Autodesk Inventor part; units mm, degrees
ref_plane "YZ Plane" through (0, 0, 0) normal (1, 0, 0) x (0, 1, 0)
ref_plane "XZ Plane" through (0, 0, 0) normal (0, 1, 0) x (-1, 0, 0)
ref_plane "XY Plane" through (0, 0, 0) normal (0, 0, 1) x (1, 0, 0)
sketch "Sketch1" plane through (0, 0, 0) normal (1, 0, 0) x (0, 1, 0)
  line L0 (0, 0) -> (50, 0)
  line L1 (50, 0) -> (50, 20)
  line L2 (50, 20) -> (0, 20)
  line L3 (0, 20) -> (0, 0)
  dimension "d0" = 50
  dimension "d1" = 20
extrude "Extrusion1" add sketch "Sketch1" along normal blind 5
sketch "Sketch2" plane through (5, 0, 0) normal (1, 0, 0) x (0, 0, -1)
  line L0 (-20, 50) -> (-20, 0)
  line L1 (-20, 25) -> (0, 25)
  line L2 (0, 0) -> (0, 50)
  line L3 (-20, 20) -> (0, 20)
  line L4 (0, 50) -> (-20, 50) construction
  line L5 (-10, 50) -> (-10, 0) construction
  line L6 (-20, 0) -> (0, 0) construction
  circle A0 centre (-10, 37.5) radius 2.6
  circle A1 centre (-10, 12.5) radius 2.6
  circle A2 centre (-10, 37.5) radius 4.625 construction
  circle A3 centre (-10, 12.5) radius 4.625 construction
  line L7 (-20, 25) -> (-16.5, 25)
  line L8 (-16.5, 25) -> (-16.5, 50)
  line L9 (-16.5, 50) -> (-20, 50)
  line L10 (-20, 50) -> (-20, 25)
  line L11 (0, 25) -> (-3.5, 25)
  line L12 (-3.5, 25) -> (-3.5, 50)
  line L13 (-3.5, 50) -> (0, 50)
  line L14 (0, 50) -> (0, 25)
  line L15 (-20, 20) -> (-16.5, 20)
  line L16 (-16.5, 20) -> (-16.5, 0)
  line L17 (-16.5, 0) -> (-20, 0)
  line L18 (-20, 0) -> (-20, 20)
  line L19 (0, 20) -> (-3.5, 20)
  line L20 (-3.5, 20) -> (-3.5, 0)
  line L21 (-3.5, 0) -> (0, 0)
  line L22 (0, 0) -> (0, 20)
  dimension "d4" = 5
  dimension "d5" = 5.2
  dimension "d6" = 5.2
  dimension "d7" = 12.5
  dimension "d8" = 12.5
  dimension "d9" = 9.25
  dimension "d10" = 9.25
  dimension "d11" = 3.5
  dimension "d12" = 3.5
  dimension "d13" = 3.5
  dimension "d14" = 3.5
extrude "Extrusion2" add sketch "Sketch2" along normal blind 49 contours L9 L8 L1 L0 | L1 L2 L3 L0 | L3 L16 L17 L0 | L12 L13 L2 L1 | L3 L2 L21 L20
chamfer "Chamfer1" distance 25 distance2 27 1 edges at (54, 50, 1.75) measured on face at (54, 23.3333, 18.8333)
chamfer "Chamfer2" distance 25 distance2 27 1 edges at (54, 50, 18.25) measured on face at (54, 23.3333, 18.8333)
chamfer "Chamfer3" distance 20 distance2 27 1 edges at (54, 0, 18.25) measured on face at (54, 15, 18.8333)
chamfer "Chamfer4" distance 20 distance2 27 1 edges at (54, 0, 1.75) measured on face at (54, 15, 1.1667)
sketch "Sketch3" plane through (54, 0, 0) normal (1, 0, 0) x (0, 0, -1)
  line L0 (0, 20) -> (-3.5, 20)
  line L1 (0, 20) -> (0, 25)
  line L2 (-3.5, 25) -> (0, 25)
  line L3 (-3.5, 25) -> (-16.5, 25)
  line L4 (-20, 25) -> (-16.5, 25)
  line L5 (-20, 25) -> (-20, 20)
  line L6 (-16.5, 20) -> (-20, 20)
  line L7 (-16.5, 20) -> (-3.5, 20)
  point P0 (0, 0)
extrude "Extrusion3" add sketch "Sketch3" along normal blind 83
sketch "Sketch4" plane through (5, 25, 16.5) normal (0, 1, 0) x (1, 0, 0)
  line L0 (132, -3.5) -> (132, 16.5)
  line L1 (132, 9) -> (34, 9)
  line L2 (34, 9) -> (34, 4)
  line L3 (34, 4) -> (132, 4)
  line L4 (132, 4) -> (132, 9)
  line L5 (49, 16.5) -> (132, 16.5)
  point P0 (-5, 16.5)
  dimension "d31" = 98
  dimension "d32" = 5
  dimension "d33" = 7.5
extrude "Extrusion4" add sketch "Sketch4" along normal blind 5
sketch "Sketch5" plane through (5, 20, 3.5) normal (0, -1, 0) x (1, 0, 0)
  line L0 (34, 9) -> (34, 4)
  line L1 (132, 9) -> (34, 9)
  line L2 (34, 4) -> (132, 4)
  line L3 (132, 16.5) -> (132, -3.5)
  point P0 (-5, -3.5)
extrude "Extrusion5" add sketch "Sketch5" along normal blind 5
chamfer "Chamfer5" distance 15 distance2 5 1 edges at (137, 30, 10) measured on face at (104.3333, 30, 10.8333)
chamfer "Chamfer6" distance 15 distance2 5 1 edges at (39, 30, 10) measured on face at (94.3333, 30, 10.8333)
chamfer "Chamfer7" distance 15 distance2 5 1 edges at (137, 15, 10) measured on face at (104.3333, 15, 9.1667)
chamfer "Chamfer8" distance 15 distance2 5 1 edges at (39, 15, 10) measured on face at (94.3333, 15, 9.1667)
sketch "Sketch6" plane through (5, 0, 0) normal (1, 0, 0) x (0, 0, -1)
  line L0 (-3.5, 50) -> (-16.5, 50) construction
  line L1 (-10, 50) -> (-10, 0) construction
  line L2 (-20, 0) -> (0, 0) construction
  circle A0 centre (-10, 37.5) radius 2.6
  circle A1 centre (-10, 12.5) radius 2.6
  dimension "d50" = 5.2
  dimension "d51" = 5.2
  dimension "d52" = 12.5
  dimension "d53" = 12.5
extrude "Extrusion6" cut sketch "Sketch6" against normal up to next
sketch "Sketch7" plane through (0, 0, 20) normal (0, 0, 1) x (1, 0, 0)
  line L0 (39, 20) -> (137, 20)
  line L1 (39, 25) -> (137, 25)
  line L2 (137, 20) -> (73, 20)
  line L3 (73, 20) -> (73, 25)
  line L4 (73, 25) -> (137, 25)
  line L5 (137, 25) -> (137, 20)
  point P0 (0, 0)
  point P1 (73, 20)
  dimension "d56" = 64
extrude "Extrusion7" add sketch "Sketch7" along normal blind 20.7
sketch "Sketch8" plane through (5, 25, 16.5) normal (0, 1, 0) x (1, 0, 0)
  line L0 (68, -3.5) -> (68, -24.2)
  line L1 (68, -24.2) -> (132, -24.2)
  line L2 (132, -24.2) -> (132, 3.8)
  line L3 (132, 3.8) -> (68, 3.8)
  line L4 (68, 3.8) -> (68, -24.2)
  line L5 (72, -20.7) -> (128, -20.7) construction
  line L6 (128, -20.7) -> (128, 0.3) construction
  line L7 (128, 0.3) -> (72, 0.3) construction
  line L8 (72, 0.3) -> (72, -20.7) construction
  circle A0 centre (72, -20.7) radius 2.6
  circle A1 centre (72, 0.3) radius 2.6
  circle A2 centre (128, -20.7) radius 2.6
  circle A3 centre (128, 0.3) radius 2.6
  point P0 (-5, 16.5)
  dimension "d59" = 64
  dimension "d60" = 28
  dimension "d61" = 56
  dimension "d62" = 21
  dimension "d63" = 3.5
  dimension "d64" = 4
  dimension "d65" = 5.2
  dimension "d66" = 5.2
  dimension "d67" = 5.2
  dimension "d68" = 5.2
extrude "Extrusion8" cut sketch "Sketch8" against normal up to next contours A0 | A1 | A2 | A3
sketch "Sketch9" plane through (5, 20, 3.5) normal (0, -1, 0) x (1, 0, 0)
  line L0 (68, 37.2) -> (132, 37.2)
  line L1 (117, 9) -> (49, 9)
  line L2 (102.5, 37.2) -> (97.5, 37.2)
  line L3 (97.5, 37.2) -> (97.5, 9)
  line L4 (97.5, 9) -> (102.5, 9)
  line L5 (102.5, 9) -> (102.5, 37.2)
  line L6 (132, 9) -> (132, 37.2)
  point P0 (-5, -3.5)
  point P1 (102.5, 9)
  dimension "d71" = 5
  dimension "d72" = 29.5
extrude "Extrusion9" add sketch "Sketch9" along normal blind 5
chamfer "Chamfer9" distance 15 distance2 5 1 edges at (105, 15, 40.7) measured on face at (92.8333, 15, 9.1667)
chamfer "Chamfer10" distance 15 angle 45 4 edges at (27, 50, 18.25) (27, 50, 1.75) (27, 0, 1.75) (27, 0, 18.25)
chamfer "Chamfer11" distance 20.7 angle 45 1 edges at (73, 22.5, 20)
equation "\"d8\" = d7"
equation "\"d10\" = d9"
equation "\"d53\" = d52"
equation "\"d54\" = d51"
properties part number "Y Axis Limit Switch Mount"
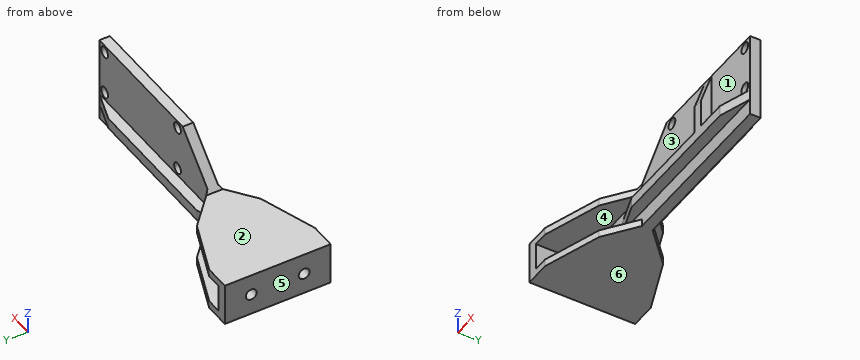
Check sheet for the modelled part. Datum: model origin and axes. Units: mm. Face numbers are marked on the shaded views. A direction names the side the tool comes from. Round coordinates to 2 decimals unless told otherwise and drop trailing zeros. Loops run counter-clockwise (first coordinate to the right, second up) from the corner with the lowest first, then second, coordinate; pieces in that order, holes last. Notation, with made-up numbers: (37.5, -34) - (52.5, -34) arc R13 ccw to (52.5, -21) - close; hole circle Ø8 at (18.25, 46.25). An arc over 180 degrees is marked (long way). Write item = value, one per line. Start each with the question number.
Q1. Section check D-D (y = 23.5). Record the boundary of the cut face in (x, z), plus the area to 3 significant figures.
Q2. Thickness scan on L1, parallel to X at y = 23.65, z = 16.2; L2, parallel to Z at x = 77, y = 21.65; L3, parallel to Z at x = 19.5, y = 46.5. Record the ranges inside material, lowest first.
Q3. Section check B-B (z = 10). Count the separate pieces of the cut face and the enclosed holes in it, plus the area to 3 significant figures.
Q4. Depth check by flat-ended pin: P1, Ø1.5, axis at y = 18, z = 22, coming from the -X side; P2, Ø7.5, axis at x = 21.5, y = 42.5, coming from the +Z side; P3, Ø4, axis at x = 70, y = 23.5, coming from the +Z side; P4, Ø4.5, axis at x = 133, z = 16.2, coming from the +Y side. Enter the tip coordinate at first touch or a pass-through.
Q5. Section check A-A (x = 77). Record the boundary of the cut face in (y, z).
Q6. Access from +Z, -Z, +X, -X, +Y, -Y to the whole of each face (thin tool, end or side, straight path). Record for the marked faces 1 and 2.
Q7. Release check for a two-part mould opening along Z. For the marked faces 3, 4, 5 and 6 record: pulls with the +Z half, pulls with the -Z half, needs draft (parallel to the pull), parting line crosses it, or undercut.
Q8. Section check C-C (y = 37.5). Record the boundary of the cut face in (x, z), plus the area to 4 significant figures.
Derived:
q1.outline = (0, 0) - (137, 0) - (137, 40.7) - (73, 40.7) - (52.3, 20) - (0, 20) - close; hole circle Ø5.2 at (77, 16.2); hole circle Ø5.2 at (77, 37.2); hole circle Ø5.2 at (133, 16.2); hole circle Ø5.2 at (133, 37.2)
q1.area = 4,190 mm^2
q2.L1 = 0 to 74.4, 79.6 to 130.4, 135.6 to 137
q2.L2 = 0 to 13.6, 18.8 to 34.6, 39.8 to 40.7
q2.L3 = 0 to 3.5, 16.5 to 20
q3.separate_pieces = 3
q3.enclosed_holes = 0
q3.area = 1,690 mm^2
q4.P1 = 102.5
q4.P2 = 20
q4.P3 = 39.7
q4.P4 = through
q5.outline = (15, 7.5) - (20, 7.5) - (20, 0) - (25, 0) - (25, 7.5) - (30, 7.5) - (30, 12.5) - (25, 12.5) - (25, 13.6) - (20, 13.6) - (20, 12.5) - (15, 12.5) - close; (20, 18.8) - (25, 18.8) - (25, 34.6) - (20, 34.6) - close; (20, 39.8) - (25, 39.8) - (25, 40.7) - (20, 40.7) - close
q6.face_1 = +Z, +X, -Y
q6.face_2 = +Z, -X, +Y, -Y
q7.face_3 = undercut
q7.face_4 = undercut
q7.face_5 = needs draft
q7.face_6 = pulls with the -Z half
q8.outline = (0, 0) - (40.5, 0) - (40.5, 3.5) - (5, 3.5) - (5, 7.4) - (0, 7.4) - close; (0, 12.6) - (5, 12.6) - (5, 16.5) - (40.5, 16.5) - (40.5, 20) - (0, 20) - close
q8.area = 322.5 mm^2
